Model file for the job. Use its own axes, mm. Face numbers are marked on the shaded views. A direction names the side the tool comes from. Round coordinates to 2 decimals unless told otherwise and drop trailing zeros. Order: outer loops, then holes, each group sorted by start corner. A loop starts at its lowest first (then second) coordinate and runs counter-clockwise, first axis right, second up. Notation, with made-up numbers: (64.25, -14.75) -> (101.25, -14.75) arc R11 cw to (101.25, -4.75) -> close; hole circle Ø9 at (-39.5, 18.25). An arc over 180 degrees is marked (long way). Answer as CSV lines item,"result".
```python
from build123d import *

# Parameters (mm, degrees)
SKETCH2_W           = 50
SKETCH2_H           = 30
BOSS_EXTRUDE2_DEPTH = 100
CUT_EXTRUDE1_DEPTH  = 95
SKETCH4_W           = 20
SKETCH4_H           = 5
BOSS_EXTRUDE3_DEPTH = 10
BOSS_EXTRUDE4_DEPTH = 5
SKETCH6_R           = 2.55
CUT_EXTRUDE2_DEPTH  = 5
SKETCH9_R           = 2.55
BOSS_EXTRUDE6_DEPTH = 5
FILLET1_R           = 5
FILLET3_R           = 1


with BuildPart() as part:
    # Sketch2 → Boss-Extrude2 (new body)
    with BuildSketch(Plane(origin=(0, 0, 0), x_dir=(0, 0, -1), z_dir=(1, 0, 0))):
        Rectangle(SKETCH2_W, SKETCH2_H)
    boss_extrude2 = extrude(amount=BOSS_EXTRUDE2_DEPTH)

    # Sketch3 → Cut-Extrude1 (cut)
    with BuildSketch(Plane.ZY):
        with BuildLine():
            Line((22, 15), (-22, 15))
            ThreePointArc((-22, 15), (0, -7), (22, 15))
        make_face()
    cut_extrude1 = extrude(amount=-CUT_EXTRUDE1_DEPTH, mode=Mode.SUBTRACT)

    # Mirror7: Boss-Extrude2, Cut-Extrude1 across plane
    add(boss_extrude2.mirror(Plane(origin=(0, 0, 0), x_dir=(0, 0, 1), z_dir=(1, 0, 0))))
    add(cut_extrude1.mirror(Plane(origin=(0, 0, 0), x_dir=(0, 0, 1), z_dir=(1, 0, 0))), mode=Mode.SUBTRACT)

    # Sketch4 → Boss-Extrude3 (add)
    with BuildSketch(Plane.XZ.offset(15)):
        with Locations((0, -7.75)):
            Rectangle(SKETCH4_W, SKETCH4_H)
    boss_extrude3 = extrude(amount=BOSS_EXTRUDE3_DEPTH)

    # Sketch5 → Boss-Extrude4 (add)
    with BuildSketch(Plane(origin=(0, 0, -10.25), x_dir=(-1, 0, 0), z_dir=(0, 0, -1))):
        with BuildLine():
            Line((-10, -25), (10, -25))
            ThreePointArc((10, -25), (0, -35), (-10, -25))
        make_face()
    boss_extrude4 = extrude(amount=-BOSS_EXTRUDE4_DEPTH)

    # Sketch6 → Cut-Extrude2 (cut)
    with BuildSketch(Plane(origin=(0, 0, -10.25), x_dir=(-1, 0, 0), z_dir=(0, 0, -1))):
        with Locations((0, -25)):
            Circle(SKETCH6_R)
    cut_extrude2 = extrude(amount=-CUT_EXTRUDE2_DEPTH, mode=Mode.SUBTRACT)

    # Mirror12: Boss-Extrude3, Boss-Extrude4, Cut-Extrude2 across plane
    add(boss_extrude3.mirror(Plane.XY))
    add(boss_extrude4.mirror(Plane.XY))
    add(cut_extrude2.mirror(Plane.XY), mode=Mode.SUBTRACT)

    # Sketch9 → Boss-Extrude6 (add)
    with BuildSketch(Plane(origin=(0, 0, -10.25), x_dir=(-1, 0, 0), z_dir=(0, 0, -1))):
        with BuildLine():
            Line((80, -15), (95, -15))
            Line((95, -15), (95, -17.5))
            Line((95, -17.5), (100, -17.5))
            ThreePointArc((100, -17.5), (107.5, -25), (100, -32.5))
            Line((100, -32.5), (80, -32.5))
            Line((80, -32.5), (80, -15))
        make_face()
        with Locations((100, -25)):
            Circle(SKETCH9_R, mode=Mode.SUBTRACT)
    boss_extrude6 = extrude(amount=-BOSS_EXTRUDE6_DEPTH)

    # Mirror13: Boss-Extrude6 across plane
    add(boss_extrude6.mirror(Plane.XY))

    # Fillet1
    fillet1_edges = [part.edges().sort_by_distance(p)[0] for p in [
        (100, 0, 25),
        (-100, 0, -25),
        (-100, 0, 25),
        (100, 0, -25),
    ]]
    fillet(fillet1_edges, radius=FILLET1_R)

    # Fillet3
    fillet3_edges = [part.edges().sort_by_distance(p)[0] for p in [
        (-87.5, -15, -10.25),
        (-87.5, -15, 5.25),
        (-87.5, -15, 10.25),
        (-95, -15, 7.75),
        (-80, -15, 7.75),
        (-80, -32.5, 7.75),
        (10, -15, -7.75),
        (0, -15, -5.25),
        (-10, -15, -7.75),
        (0, -15, -10.25),
        (10, -15, 7.75),
        (0, -15, 5.25),
        (-10, -15, 7.75),
        (0, -15, 10.25),
        (-95, -15, -7.75),
        (-80, -32.5, -7.75),
        (-87.5, -15, -5.25),
        (-80, -15, -7.75),
    ]]
    fillet(fillet3_edges, radius=FILLET3_R)


solid = part.part
```
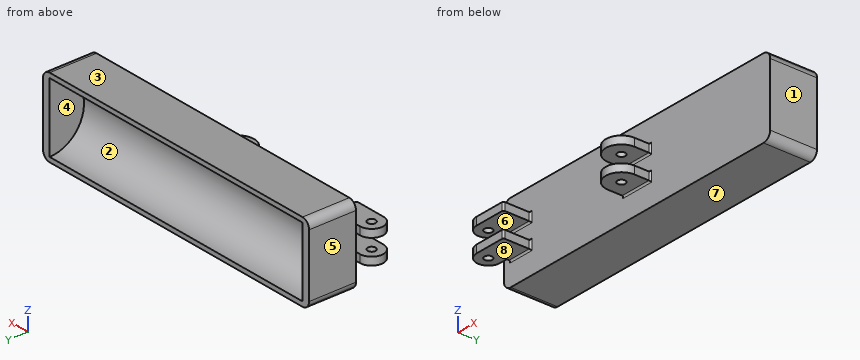
Q1. Mould opens along Z. For the marked faces 1, 2, 3 and 4 say: +Z half, -Z half, draft (parallel to the pull), parting line (faces both ways), or undercut.
Checks:
face 1,"draft"
face 2,"undercut"
face 3,"+Z half"
face 4,"undercut"
Q2. Saw through at C-C (x = 33). Write the cut outline in (y, z).
Checks:
outline,"(-15, -25) -> (15, -25) -> (15, -22) arc R22 cw to (15, 22) -> (15, 25) -> (-15, 25) -> close"
Q3. Saw through at D-D (z = 7.5). Write the cut outline in (x, y).
Checks:
outline,"(-100, -32.5) -> (-81, -32.5) arc R1 ccw to (-80, -31.5) -> (-80, -16) arc R1 cw to (-79, -15) -> (-11, -15) arc R1 cw to (-10, -16) -> (-10, -25) arc R10 ccw to (10, -25) -> (10, -16) arc R1 cw to (11, -15) -> (100, -15) -> (100, 15) -> (95, 15) -> (95, -5.68) -> (-95, -5.68) -> (-95, 15) -> (-100, 15) -> (-100, -15) -> (-96, -15) arc R1 cw to (-95, -16) -> (-95, -17.5) -> (-100, -17.5) arc R7.5 ccw to start; hole circle Ø5.1 at (-100, -25); hole circle Ø5.1 at (0, -25)"
Q4. Saw through at B-B (y = -1). Write the cut outline in (x, z).
Checks:
outline,"(-100, -20) arc R5 ccw to (-95, -25) -> (95, -25) arc R5 ccw to (100, -20) -> (100, 20) arc R5 ccw to (95, 25) -> (-95, 25) arc R5 ccw to (-100, 20) -> close; hole (-95, -15.1) -> (95, -15.1) -> (95, 15.1) -> (-95, 15.1) -> close"
Q5. Flat gauge pins, fed straight in: pin 1 (8 mm diameter, centred on x = 0, y = -25, fed in from +Z); pin 2 (4 mm diameter, centred on x = -95, z = -6.5, fed in from -Y); pin 3 (6.5 mm diameter, centred on y = 9, z = -8.5, fed in from -X). Where does each tip first touch, or does it go through?
Checks:
pin 1,"z = 10.25"
pin 2,"y = -32.5"
pin 3,"x = -100"
Q6. Wall check: L1, parallel to Z at x = -93, y = -29; L2, parallel to X at y = 12, z = -17; L3, parallel to Y at x = -80.5, z = 0.5. Give the ranges that are in metal, low to high. Write a range as [from, to].
Checks:
L1,"[-10.25, -5.25], [5.25, 10.25]"
L2,"[-100, -95], [95, 100]"
L3,"[-15, -6.99]"
Q7. Saw through at A-A (x = 0). Write the cut outline in (y, z), plus the area to 3 significant figures.
Checks:
outline,"(-35, -10.25) -> (-27.55, -10.25) -> (-27.55, -5.25) -> (-35, -5.25) -> close; (-35, 5.25) -> (-27.55, 5.25) -> (-27.55, 10.25) -> (-35, 10.25) -> close; (-22.45, -10.25) -> (-16, -10.25) arc R1 cw to (-15, -11.25) -> (-15, -25) -> (15, -25) -> (15, -22) arc R22 cw to (15, 22) -> (15, 25) -> (-15, 25) -> (-15, 11.25) arc R1 cw to (-16, 10.25) -> (-22.45, 10.25) -> (-22.45, 5.25) -> (-16, 5.25) arc R1 cw to (-15, 4.25) -> (-15, -4.25) arc R1 cw to (-16, -5.25) -> (-22.45, -5.25) -> close"
area,"890 mm²"
Q8. Tool access for the marked faces 5, 6, 7 and 8: list every direction of +Z, -Z, +X, -X, +Y, -Y with a clear straight run to the whole face (end or side of a thin tool).
Checks:
face 5,"+Z, -Z, -X, +Y"
face 6,"+X, -X, -Y"
face 7,"-Z, +X, -X, +Y, -Y"
face 8,"-Z, +X, -X, -Y"
